Here's how the part is built. I have some questions about the finished solid (model axes, mm). A direction names the side the tool comes from. Coordinates: 2 decimals unless noted, no trailing zeros. Write each loop counter-clockwise with the first axis right and the second up, starting at its lowest first coordinate (ties: lowest second). Pieces come first, ordered by that corner, then holes. Notation, with made-up numbers: (2, -26) -> (12, -26) arc R27 cw to (12, 11) -> close; hole circle Ø2 at (-19, 36.5). An arc over 180 degrees is marked (long way). Put each result on its own line as item: value. Start each with the question number.
Item 1: I want a section at A-A, the plane z = 1.8. List the corners of the cut face in (x, y) for me.
Item 2: For pin 1 (1.5 mm diameter, centred on y = -7.5, z = 1, fed in from +X), with a flat end and sliding along its axis, tell me the tip position at first contact or that it passes through.
Item 3: I want a section at B-B, the plane x = -29.5. List the corners of the cut face in (y, z) for me, then the cut area to 3 significant figures.
Item 4: On a 3-axis mill with a long thin cutter (end or side, diameter ignored), from which of +Z, -Z, +X, -X, +Y, -Y can I reach the whole of each face in a straight line? I mean faces 4 (the face through (-1, 1, 0)), 5 (the face through (-4.828, 14.208, 1.479)). Say none if no direction works.
Item 5: I want a section at C-C, the plane y = -20.5. List the corners of the cut face in (x, z) for me, then the cut area to 3 significant figures.
Item 6: I need wall thicknesses on line 1 (X direction, y = -9, z = 2.25); line 2 (X direction, y = 17, z = 1.4); line 3 (X direction, y = 10, z = 0.3). Which ranges of each line are inside material? Lowest first, please. Write a range as [from, to].
Item 7: If we mould it in two halves opening along X, with no side actions, what happens to faces 1 (the face through (2.98, 16.15, 1.48)), 2 (the face through (-1, 1, 3)), 3 (the face through (55.12, 10.44, 1.48))? For each: released by +X, released by -X, zero draft, split by the parting line, or undercut.
from build123d import *

# Parameters (mm, degrees)
PAD_DEPTH = 3


with BuildPart() as part:
    # Sketch → Pad (new body)
    with BuildSketch(Plane.XY):
        with BuildLine():
            Line((0, 0), (0, 14.502488))
            Line((0, 14.502488), (2.444644, 13.541802))
            Line((2.444644, 13.541802), (3.525413, 18.825575))
            Line((3.525413, 18.825575), (6.167308, 9.459041))
            Line((6.167308, 9.459041), (10.250262, 9.218303))
            ThreePointArc((10.250262, 9.218303), (18.202038, 12.211905), (21.296978, 20.124789))
            Line((21.296978, 20.124789), (75, 20.124789))
            ThreePointArc((75, 20.124789), (54.90279, 10.195186), (47.700768, -11.032761))
            ThreePointArc((47.700768, -11.032761), (20.35465, -12.880568), (0, -31.235753))
            Line((0, -31.235753), (0, 0))
        make_face()
    pad = extrude(amount=PAD_DEPTH)

    # Mirrored: Pad across Sketch V_Axis
    add(pad.mirror(Plane(origin=(0, 0, 0), x_dir=(0, 0, 1), z_dir=(1, 0, 0))))


solid = part.part
Calculated:
1. outline: (-75, 20.12) arc R29.31 cw to (-47.7, -11.03) arc R41.9 cw to (0, -31.24) arc R41.9 cw to (47.7, -11.03) arc R29.31 cw to (75, 20.12) -> (21.3, 20.12) arc R10.44 cw to (10.25, 9.22) -> (6.17, 9.46) -> (3.53, 18.83) -> (2.44, 13.54) -> (0, 14.5) -> (-2.44, 13.54) -> (-3.53, 18.83) -> (-6.17, 9.46) -> (-10.25, 9.22) arc R10.44 cw to (-21.3, 20.12) -> close
2. pin 1: stops at x = 47.73
3. outline: (-10.19, 0) -> (20.12, 0) -> (20.12, 3) -> (-10.19, 3) -> close
3. area: 90.9 mm2
4. face 4: -Z, +X, -X, +Y, -Y
4. face 5: +Z, -Z, +Y
5. outline: (-8.47, 0) -> (8.47, 0) -> (8.47, 3) -> (-8.47, 3) -> close
5. area: 50.8 mm2
6. line 1: x = [-47.64, 47.64]
6. line 2: x = [-63.65, -20.97], [-4.04, -3.15], [3.15, 4.04], [20.97, 63.65]
6. line 3: x = [-54.73, -14.87], [-6.01, 6.01], [14.87, 54.73]
7. face 1: undercut
7. face 2: zero draft
7. face 3: released by +X
